For this review, use the dimensioned drawing (mm, ordinates from the lowest corner) and the shaded views. A direction names the side the tool comes from. Coordinates: 2 decimals unless noted, no trailing zeros. Write each loop counter-clockwise with the first axis right and the second up, starting at its lowest first coordinate (ties: lowest second). Pieces come first, ordered by that corner, then holes. Notation, with made-up numbers: (25.25, 30) - (83.25, 30) arc R17 cw to (83.25, 50) - close; hole circle Ø11 at (-21, 59). An arc over 180 degrees is marked (long way). Use one line per item in the form item = value. Start each with the question number.
1) We need section D-D (z = 1.25). Give the boundary of the cut face in (x, y).
2) We need section A-A (z = 11). Give the boundary of the cut face in (x, y), plus the area to 3 significant figures.
3) For L1, parallel to X at y = 4, z = 4.25; L2, parallel to Z at x = 37.5, y = 6.5; L3, parallel to X at y = 5, z = 2.75, list the stretches that pass through material, from the lowest coordinate up. Write a range as from..to.
4) We need section B-B (y = 6.25). Count the separate pieces of the cut face and the enclosed holes in it, plus the area to 3 significant figures.
5) Insertion check: P1, Ø1.5, axis at x = 29.5, y = 7, coming from the -Z side; P2, Ø1.7, axis at x = 6, y = 3.5, coming from the +Z side; P3, Ø2.5, axis at x = 18, y = 4, coming from the -Z side. Each pin has a flat end and moves straight along its axis. Give the tip position at first contact, or say it passes through.
6) Tool access review of the marked faces 1, 2, 3 and 4: name each direction out of +Z, -Z, +X, -X, +Y, -Y from which nothing blocks a thin tool from reaching the whole face with its end or side.
7) We need section C-C (z = 7). Give the boundary of the cut face in (x, y), plus the area to 3 significant figures.
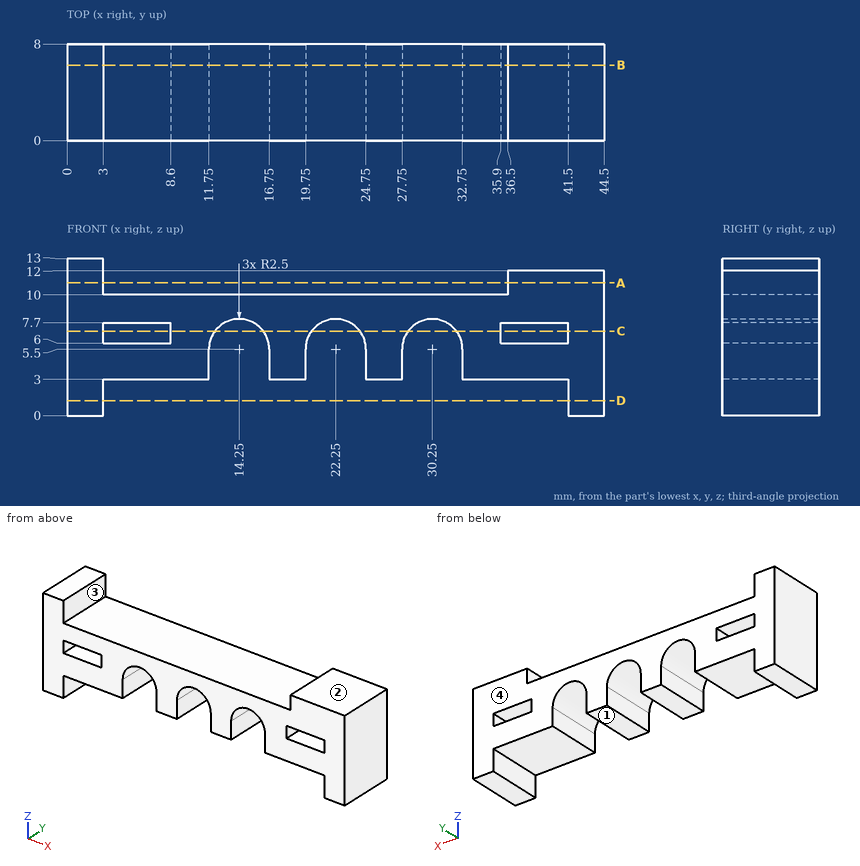
Determined:
q1.outline = (0, 0) - (3, 0) - (3, 8) - (0, 8) - close; (41.5, 0) - (44.5, 0) - (44.5, 8) - (41.5, 8) - close
q2.outline = (0, 0) - (3, 0) - (3, 8) - (0, 8) - close; (36.5, 0) - (44.5, 0) - (44.5, 8) - (36.5, 8) - close
q2.area = 88.0 mm²
q3.L1 = 0..11.75, 16.75..19.75, 24.75..27.75, 32.75..44.5
q3.L2 = 3..6, 7.7..12
q3.L3 = 0..3, 41.5..44.5
q4.separate_pieces = 1
q4.enclosed_holes = 2
q4.area = 269 mm²
q5.P1 = 7.5
q5.P2 = 10
q5.P3 = 3
q6.face_1 = -Z, +Y, -Y
q6.face_2 = +Z, +X, +Y, -Y
q6.face_3 = +Z, +Y, -Y
q6.face_4 = +Z, -Z, +X, -X, +Y
q7.outline = (0, 0) - (3, 0) - (3, 8) - (0, 8) - close; (8.6, 0) - (12.25, 0) - (12.25, 8) - (8.6, 8) - close; (16.25, 0) - (20.25, 0) - (20.25, 8) - (16.25, 8) - close; (24.25, 0) - (28.25, 0) - (28.25, 8) - (24.25, 8) - close; (32.25, 0) - (35.9, 0) - (35.9, 8) - (32.25, 8) - close; (41.5, 0) - (44.5, 0) - (44.5, 8) - (41.5, 8) - close
q7.area = 170 mm²
